Can you work these out from the drawing? Everything is in mm from the part's minimum corner. Round coordinates to 2 decimals unless told otherwise and drop trailing zeros. Loops run counter-clockwise (first coordinate to the right, second up) from the corner with the lowest first, then second, coordinate; pieces in that order, holes last. Notation, with made-up numbers: M 71,29.5 L 97,29.5 A18 cw 97,54.5 Z; hole C 67,36 d11. An arc over 180 degrees is marked long. Use a Markdown table: item, result.
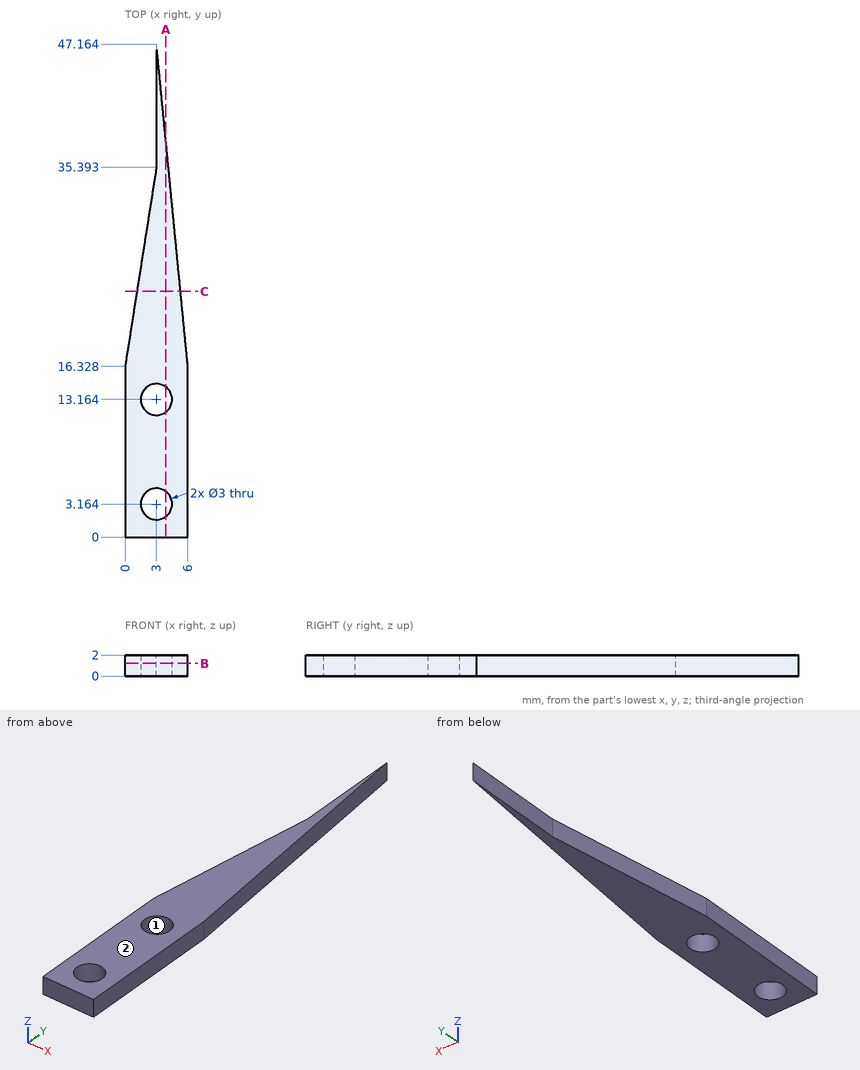
1. Imagine slicing it at A-A, the plane x = 3.9. Write out the boundary of the cut face in (y, z).
Answer sheet:
| item | result |
|---|---|
| outline | M 0,0 L 1.96,0 L 1.96,2 L 0,2 Z; M 4.36,0 L 11.96,0 L 11.96,2 L 4.36,2 Z; M 14.36,0 L 37.91,0 L 37.91,2 L 14.36,2 Z |
2. Imagine slicing it at C-C, the plane y = 23.5. Write out the boundary of the cut face in (x, z).
Answer sheet:
| item | result |
|---|---|
| outline | M 1.13,0 L 5.3,0 L 5.3,2 L 1.13,2 Z |
3. Imagine slicing it at B-B, the plane z = 1.2. Write out the boundary of the cut face in (x, y), then the cut area to 3 significant figures.
Answer sheet:
| item | result |
|---|---|
| outline | M 0,0 L 6,0 L 6,16.33 L 3,47.16 L 3,35.39 L 0,16.33 Z; hole C 3,3.16 d3; hole C 3,13.16 d3 |
| area | 159 mm2 |
4. We'd pull the mould along X, two halves only. Please class the marked faces 1 and 2: +X half, -X half, draft (parallel to the pull), parting line (faces both ways), or undercut.
Answer sheet:
| item | result |
|---|---|
| face 1 | undercut |
| face 2 | draft |
5. I need wall thicknesses on probe 1 along X at (y, z) = (3, 0.7); probe 2 along X at (y, z) = (12, 0.8) (1 decimal); probe 3 along X at (y, z) = (30, 1.2). Which ranges of each line are inside material? Lowest first, please. Write a range as from..to.
Answer sheet:
| item | result |
|---|---|
| probe 1 | 0..1.51, 4.49..6 |
| probe 2 | 0..2.1, 3.9..6 |
| probe 3 | 2.15..4.67 |
